Input: part model. Units: mm. Frame: model coordinates. Face numbers are marked on the shaded views. Give positions to 0.01 mm unless a question says otherwise; leave off trailing zeros. Loops run counter-clockwise (first coordinate to the right, second up) from the corner with the lowest first, then second, coordinate; pieces in that order, holes last.
Autodesk Inventor part; units mm, degrees
ref_plane "YZ Plane" through (0, 0, 0) normal (1, 0, 0) x (0, 1, 0)
ref_plane "XZ Plane" through (0, 0, 0) normal (0, 1, 0) x (-1, 0, 0)
ref_plane "XY Plane" through (0, 0, 0) normal (0, 0, 1) x (1, 0, 0)
sketch "Sketch1" plane through (0, 0, 0) normal (0, 1, 0) x (-1, 0, 0)
  line L0 (-15, 15) -> (15, 15)
  line L1 (15, 15) -> (15, -15)
  line L2 (15, -15) -> (-15, -15)
  line L3 (-15, -15) -> (-15, 15)
  line L4 (-15, 15) -> (15, -15) construction
  line L5 (15, 15) -> (-15, -15) construction
  line L6 (15, -10) -> (-15, -15)
  line L7 (21, 0) -> (-21, 0) construction
  line L8 (15, 10) -> (-15, 15)
  point P0 (0, 0)
  point P1 (0, 0)
  point P2 (-15, 15)
  point P3 (15, 10)
  dimension "d1" = 30
  dimension "d2" = 30
  dimension "d19" = 20
  dimension "d20" = 30
extrude "Extrusion1" add sketch "Sketch1" against normal blind 8 contours L8 L1 L6 L3
hole "Hole1" at (0, 0, 0) direction (0, -1, 0) diameter 3 end through all countersink diameter 3.5 countersink angle 90
chamfer "Chamfer1" distance 0.25 angle 45 1 edges at (0, -8, -1.5)
fillet "Fillet1" radius 5 2 edges at (-15, -4, 10) (-15, -4, -10)
chamfer "Chamfer3" distance 4 angle 45 1 edges at (15, -8, 0)
properties part number "TCSM1-002A" material "Wood (Oak)"
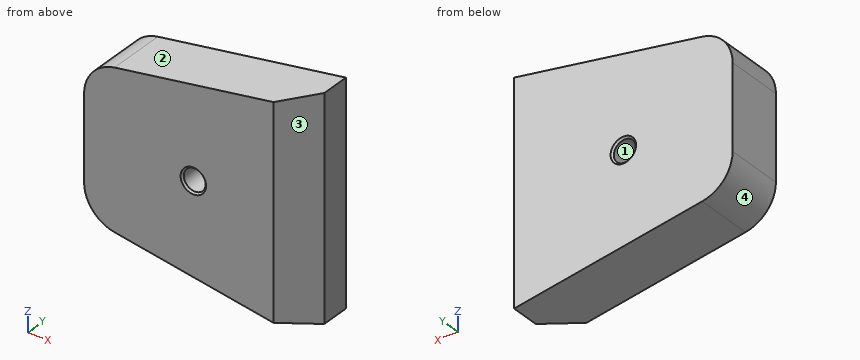
(1) Cut plane C-C (y = -6.5). Return the cut outline in (x, z), and give its area (3 significant figures).
Values follow:
outline: (-15, -5.76) arc R5 ccw to (-10.82, -10.7) - (12.5, -14.58) - (12.5, 14.58) - (-10.82, 10.7) arc R5 ccw to (-15, 5.76) - close; hole circle Ø3 at (0, 0)
area: 662 mm2
(2) Cut plane D-D (z = 12). Return the cut outline in (x, y), and give its area (3 significant figures).
Values follow:
outline: (-3, -8) - (11, -8) - (15, -4) - (15, 0) - (-3, 0) - close
area: 136 mm2
(3) Cut plane B-B (x = 0). Return the cut outline in (y, z), and give its area (3 significant figures).
Values follow:
outline: (-8, -12.5) - (0, -12.5) - (0, -1.75) - (-0.25, -1.5) - (-7.75, -1.5) - (-8, -1.75) - close; (-8, 1.75) - (-7.75, 1.5) - (-0.25, 1.5) - (0, 1.75) - (0, 12.5) - (-8, 12.5) - close
area: 176 mm2
(4) Cut plane A-A (z = 0). Return the cut outline in (x, y), and give its area (3 significant figures).
Values follow:
outline: (-15, -8) - (-1.75, -8) - (-1.5, -7.75) - (-1.5, -0.25) - (-1.75, 0) - (-15, 0) - close; (1.5, -7.75) - (1.75, -8) - (11, -8) - (15, -4) - (15, 0) - (1.75, 0) - (1.5, -0.25) - close
area: 208 mm2
(5) Mould query, pull axis Z, two halves, no side actions, for the marked faces 1, 2, 3 and 4. Classes: +Z half, -Z half, draft (parallel to the pull), parting line (faces both ways), or undercut.
Values follow:
face 1: undercut
face 2: +Z half
face 3: draft
face 4: -Z half
(6) Ray query, probe 1 along X at (y, z) = (-3.5, 0); probe 2 along Z at (x, y) = (0, -2.5); probe 3 along X at (y, z) = (-4.5, 0). Return the intervals inside material, ascending.
Values follow:
probe 1: x = -15 to -1.5, 1.5 to 15
probe 2: z = -12.5 to -1.5, 1.5 to 12.5
probe 3: x = -15 to -1.5, 1.5 to 14.5
(7) Pin query (flat end, axial travel): pin 1 Ø3 at (x, y) = (5, -4) entering from -Z; pin 2 Ø3 at (y, z) = (-4, -11.5) entering from -X; pin 3 Ø3 at (x, y) = (-6, -5) entering from -Z. Return the tip coordinate at first contact, or that it passes through.
Values follow:
pin 1: stops at z = -13.58
pin 2: stops at x = -12.66
pin 3: stops at z = -11.75
